Input: part model. Units: mm. Frame: model coordinates. Round coordinates to 2 decimals unless told otherwise and drop trailing zeros. Loops run counter-clockwise (first coordinate to the right, second up) from the corner with the lowest first, then second, coordinate; pieces in that order, holes last. Notation, with made-up numbers: (13, -15.75) - (54, -15.75) arc R16 ccw to (54, -3.75) - close; hole circle Ø11 at (50, 40). An arc over 180 degrees is marked (long way). One line per question, with ' | ' between items. Start each with the question number.
Item 1: First-contact query: pin 1 (2 mm diameter, centred on y = -12.5, z = 2, fed in from -X); pin 2 (5 mm diameter, centred on x = -30.5, y = -35.5, fed in from +Z); pin 3 (2 mm diameter, centred on x = 9.5, z = 2, fed in from -Y). Flat tips, straight axial feed; report the tip coordinate or a pass-through.
Item 2: Section B-B, the plane y = 57. Return loops of the section in (x, z), plus the area to 3 significant figures.
Item 3: Material intervals for line 1 along Y through (x, z) = (0, 1.4); line 2 along Z through (x, y) = (-62, 4); line 3 along X through (y, z) = (-58, 1.8), sorted ascending.
Item 4: Draft query along Y for faces 1 (the face through (-1, 1, 0)), 2 (the face through (68.86, 21.69, 2.96)), 3 (the face through (-1, 1, 5)), 4 (the face through (-53.57, -41.07, 5.51)). Return one class per face: pulls with the +Y half, pulls with the -Y half, needs draft (parallel to the pull), parting line crosses it, or undercut.
Item 5: Section C-C, the plane y = 0. Return loops of the section in (x, z), plus the area to 3 significant figures.
Item 6: Section A-A, the plane x = 0. Return loops of the section in (y, z).
Item 7: Section D-D, the plane z = 1.95. Return loops of the section in (x, y).
```python
from build123d import *

# Parameters (mm, degrees)
F0_R     = 24.06525
F0_R_2   = 1.05
F1_DEPTH = 2
F2_SIZE  = 1
F3_SCALE = 3
F4_R     = 67.5
F5_DEPTH = 1


with BuildPart() as f1:
    # F0 (on Top) → F1 (new body)
    with BuildSketch(Plane.XY):
        Circle(F0_R)
        with Locations((0, -19)):
            Circle(F0_R_2, mode=Mode.SUBTRACT)
        with Locations((0, 19)):
            Circle(F0_R_2, mode=Mode.SUBTRACT)
    extrude(amount=F1_DEPTH)

    # F2
    f2_edges = [f1.edges().sort_by_distance(p)[0] for p in [
        (-1.05, 19, 2),
        (-1.05, -19, 2),
    ]]
    chamfer(f2_edges, length=F2_SIZE)


with BuildPart() as f1_1:
    # F3: moved
    add(f1.part.scale(F3_SCALE))

    # F4 (on face) → F5 (cut)
    with BuildSketch(Plane.XY.offset(6)):
        Circle(F4_R)
    extrude(amount=-F5_DEPTH, mode=Mode.SUBTRACT)


solid = f1_1.part
```
Return value:
1) pin 1: x = -71.27 | pin 2: z = 5 | pin 3: y = -71.69
2) outline: (-44.31, 0) - (-3.15, 0) - (-3.15, 3) - (-5.15, 5) - (-36.16, 5) - (-36.16, 6) - (-44.31, 6) - close; (3.15, 0) - (44.31, 0) - (44.31, 6) - (36.16, 6) - (36.16, 5) - (5.15, 5) - (3.15, 3) - close | area: 424 mm2
3) line 1: -72.2 to -60.15, -53.85 to 53.85, 60.15 to 72.2 | line 2: 0 to 5 | line 3: -42.99 to -2.99, 2.99 to 42.99
4) face 1: needs draft | face 2: parting line crosses it | face 3: undercut | face 4: undercut
5) outline: (-72.2, 0) - (72.2, 0) - (72.2, 6) - (67.5, 6) - (67.5, 5) - (-67.5, 5) - (-67.5, 6) - (-72.2, 6) - close | area: 731 mm2
6) outline: (-72.2, 0) - (-60.15, 0) - (-60.15, 3) - (-62.15, 5) - (-67.5, 5) - (-67.5, 6) - (-72.2, 6) - close; (-53.85, 0) - (53.85, 0) - (53.85, 3) - (51.85, 5) - (-51.85, 5) - (-53.85, 3) - close; (60.15, 0) - (72.2, 0) - (72.2, 6) - (67.5, 6) - (67.5, 5) - (62.15, 5) - (60.15, 3) - close
7) outline: circle Ø144.39 at (0, 0); hole circle Ø6.3 at (0, -57); hole circle Ø6.3 at (0, 57)
